```python
from build123d import *

# Parameters (mm, degrees)
ACTUATOR_HOUSING_MOUNT_R    = 64.3
ACTUATOR_HOUSING_MOUNT_R_2  = 55.8
ACTUATOR_HOUSING_MOUNT_R_3  = 1.6
ACTUATOR_HOUSING_WALL_DEPTH = 25
SKETCH2_R                   = 64.3
SKETCH2_R_2                 = 1.6
SKETCH2_R_3                 = 55.8
BOSS_EXTRUDE2_DEPTH         = 5
CUT_EXTRUDE1_START          = -5
SKETCH3_R                   = 11.45
CUT_EXTRUDE1_DEPTH          = 4
SKETCH4_R                   = 11
CUT_EXTRUDE2_DEPTH          = 4
BOSS_EXTRUDE3_START         = 8
SKETCH6_R                   = 64.3
SKETCH6_R_2                 = 63.1
BOSS_EXTRUDE3_DEPTH         = 8
SKETCH7_R                   = 1.95
M3_INSERT_L12_DEPTH         = 12
CHAMFER2_SIZE               = 0.5
SKETCH9_R                   = 1.95
CUT_EXTRUDE5_DEPTH          = 10


with BuildPart() as part:
    # Actuator Housing Mount → Actuator Housing Wall (new body)
    with BuildSketch(Plane.XY.offset(19)):
        Circle(ACTUATOR_HOUSING_MOUNT_R)
        Circle(ACTUATOR_HOUSING_MOUNT_R_2, mode=Mode.SUBTRACT)
        with Locations((57.375994082, 15.373851279)):
            Circle(ACTUATOR_HOUSING_MOUNT_R_3, mode=Mode.SUBTRACT)
        with Locations((57.375994082, -15.373851279)):
            Circle(ACTUATOR_HOUSING_MOUNT_R_3, mode=Mode.SUBTRACT)
        with Locations((42.002142802, -42.002142802)):
            Circle(ACTUATOR_HOUSING_MOUNT_R_3, mode=Mode.SUBTRACT)
        with Locations((15.373851279, -57.375994082)):
            Circle(ACTUATOR_HOUSING_MOUNT_R_3, mode=Mode.SUBTRACT)
        with Locations((-15.373851279, -57.375994082)):
            Circle(ACTUATOR_HOUSING_MOUNT_R_3, mode=Mode.SUBTRACT)
        with Locations((-42.002142802, -42.002142802)):
            Circle(ACTUATOR_HOUSING_MOUNT_R_3, mode=Mode.SUBTRACT)
        with Locations((-57.375994082, -15.373851279)):
            Circle(ACTUATOR_HOUSING_MOUNT_R_3, mode=Mode.SUBTRACT)
        with Locations((-57.375994082, 15.373851279)):
            Circle(ACTUATOR_HOUSING_MOUNT_R_3, mode=Mode.SUBTRACT)
        with Locations((-42.002142802, 42.002142802)):
            Circle(ACTUATOR_HOUSING_MOUNT_R_3, mode=Mode.SUBTRACT)
        with Locations((-15.373851279, 57.375994082)):
            Circle(ACTUATOR_HOUSING_MOUNT_R_3, mode=Mode.SUBTRACT)
        with Locations((15.373851279, 57.375994082)):
            Circle(ACTUATOR_HOUSING_MOUNT_R_3, mode=Mode.SUBTRACT)
        with Locations((42.002142802, 42.002142802)):
            Circle(ACTUATOR_HOUSING_MOUNT_R_3, mode=Mode.SUBTRACT)
    extrude(amount=-ACTUATOR_HOUSING_WALL_DEPTH)

    # Sketch2 → Boss-Extrude2 (add)
    # profile 1 of 2: a face of its own
    with BuildSketch(Plane(origin=(0, 0, -6), x_dir=(-1, 0, 0), z_dir=(0, 0, -1))):
        with Locations(Location((0, 0, 0), (0, 0, 180))):
            Circle(SKETCH2_R)
        with Locations(Location((-15.373851279, 57.375994082, 0), (0, 0, 180))):
            Circle(SKETCH2_R_2, mode=Mode.SUBTRACT)
        with Locations(Location((42.002142802, 42.002142802, 0), (0, 0, 180))):
            Circle(SKETCH2_R_2, mode=Mode.SUBTRACT)
        with Locations(Location((57.375994082, -15.373851279, 0), (0, 0, 180))):
            Circle(SKETCH2_R_2, mode=Mode.SUBTRACT)
        with Locations(Location((15.373851279, -57.375994082, 0), (0, 0, 180))):
            Circle(SKETCH2_R_2, mode=Mode.SUBTRACT)
        with Locations(Location((-42.002142802, -42.002142802, 0), (0, 0, 180))):
            Circle(SKETCH2_R_2, mode=Mode.SUBTRACT)
        with Locations(Location((-57.375994082, -15.373851279, 0), (0, 0, 180))):
            Circle(SKETCH2_R_2, mode=Mode.SUBTRACT)
        with Locations(Location((-57.375994082, 15.373851279, 0), (0, 0, 180))):
            Circle(SKETCH2_R_2, mode=Mode.SUBTRACT)
        with Locations(Location((0, 0, 0), (0, 0, 180))):
            Circle(SKETCH2_R_3, mode=Mode.SUBTRACT)
        with Locations(Location((-15.373851279, -57.375994082, 0), (0, 0, 180))):
            Circle(SKETCH2_R_2, mode=Mode.SUBTRACT)
        with Locations(Location((42.002142802, -42.002142802, 0), (0, 0, 180))):
            Circle(SKETCH2_R_2, mode=Mode.SUBTRACT)
        with Locations(Location((57.375994082, 15.373851279, 0), (0, 0, 180))):
            Circle(SKETCH2_R_2, mode=Mode.SUBTRACT)
        with Locations(Location((15.373851279, 57.375994082, 0), (0, 0, 180))):
            Circle(SKETCH2_R_2, mode=Mode.SUBTRACT)
        with Locations(Location((-42.002142802, 42.002142802, 0), (0, 0, 180))):
            Circle(SKETCH2_R_2, mode=Mode.SUBTRACT)
    # profile 2 of 2: a face of its own
    with BuildSketch(Plane(origin=(0, 0, -6), x_dir=(-1, 0, 0), z_dir=(0, 0, -1))):
        with Locations(Location((0, 0, 0), (0, 0, 180))):
            Circle(SKETCH2_R_3)
    extrude(amount=BOSS_EXTRUDE2_DEPTH)

    # Sketch3 → Cut-Extrude1 (cut)
    with BuildSketch(Plane(origin=(0, 0, -11), x_dir=(-1, 0, 0), z_dir=(0, 0, -1)).offset(CUT_EXTRUDE1_START)):
        Circle(SKETCH3_R)
    extrude(amount=CUT_EXTRUDE1_DEPTH, mode=Mode.SUBTRACT)

    # Sketch4 → Cut-Extrude2 (cut)
    with BuildSketch(Plane(origin=(0, 0, -11), x_dir=(-1, 0, 0), z_dir=(0, 0, -1))):
        Circle(SKETCH4_R)
    extrude(amount=-CUT_EXTRUDE2_DEPTH, mode=Mode.SUBTRACT)

    # Sketch6 → Boss-Extrude3 (add)
    with BuildSketch(Plane.XY.offset(19).offset(BOSS_EXTRUDE3_START)):
        Circle(SKETCH6_R)
        Circle(SKETCH6_R_2, mode=Mode.SUBTRACT)
    extrude(amount=-BOSS_EXTRUDE3_DEPTH)

    # Sketch7 → M3 Insert L12 (cut)
    with BuildSketch(Plane.XY.offset(19)):
        with Locations((57.375994082, -15.373851279)):
            Circle(SKETCH7_R)
        with Locations((42.002142802, -42.002142802)):
            Circle(SKETCH7_R)
        with Locations((15.373851279, -57.375994082)):
            Circle(SKETCH7_R)
        with Locations((-15.373851279, -57.375994082)):
            Circle(SKETCH7_R)
        with Locations((-42.002142802, -42.002142802)):
            Circle(SKETCH7_R)
        with Locations((-57.375994082, -15.373851279)):
            Circle(SKETCH7_R)
        with Locations((-57.375994082, 15.373851279)):
            Circle(SKETCH7_R)
        with Locations((-42.002142802, 42.002142802)):
            Circle(SKETCH7_R)
        with Locations((-15.373851279, 57.375994082)):
            Circle(SKETCH7_R)
        with Locations((15.373851279, 57.375994082)):
            Circle(SKETCH7_R)
        with Locations((42.002142802, 42.002142802)):
            Circle(SKETCH7_R)
        with Locations((57.375994082, 15.373851279)):
            Circle(SKETCH7_R)
    extrude(amount=-M3_INSERT_L12_DEPTH, mode=Mode.SUBTRACT)

    # Chamfer2
    chamfer2_edges = [part.edges().sort_by_distance(p)[0] for p in [
        (-64.3, 0, 27),
        (-64.3, 0, -11),
    ]]
    chamfer(chamfer2_edges, length=CHAMFER2_SIZE)

    # Sketch9 → Cut-Extrude5 (cut)
    with BuildSketch(Plane(origin=(0, 0, -11), x_dir=(-1, 0, 0), z_dir=(0, 0, -1))):
        with Locations((-30, 22)):
            Circle(SKETCH9_R)
        with Locations((30, 22)):
            Circle(SKETCH9_R)
        with Locations((30, -22)):
            Circle(SKETCH9_R)
        with Locations((-30, -22)):
            Circle(SKETCH9_R)
    extrude(amount=-CUT_EXTRUDE5_DEPTH, mode=Mode.SUBTRACT)


solid = part.part
```
Build history of the part. All positions in model axes, mm. A direction names the side the tool comes from. Round coordinates to 2 decimals unless told otherwise and drop trailing zeros. Write each loop counter-clockwise with the first axis right and the second up, starting at its lowest first coordinate (ties: lowest second). Pieces come first, ordered by that corner, then holes.
1) Band-saw the part on A-A, the plane y = 0. List the corners of the cut face in (x, z).
2) 3-axis set-ups, long thin cutter, end or side, ignore diameter. For faces 1 (the cylindrical face through (-57.58, -16.96, -1.87)), 2 (the cylindrical face through (-55.516, -14.788, 13.084)): which of +Z, -Z, +X, -X, +Y, -Y reach the whole face in a straight line?
3) Band-saw the part on C-C, the plane z = 14. Give the number of separate pieces and of enclosed holes in the cut face, and give its area (3 significant figures).
4) Mould opens along Y. For faces 3 (the flat face through (13, -1, -11)), 4 (the flat face through (-1, 12, -6)) say: +Y half, -Y half, draft (parallel to the pull), parting line (faces both ways), or undercut.
5) Drill centre lines: probe 1 along Y at (x, z) = (1, 25.5); probe 2 along Z at (x, y) = (-5.5, 37); probe 3 along Y at (x, z) = (31, -5). Where is each one in solid material? Low to high.
6) Pin check, flat tips, straight feed: pin 1 (5 mm diameter, centred on x = -57.38, y = -15.37, fed in from +Z); pin 2 (8 mm diameter, centred on y = -32, z = -7, fed in from +X); pin 3 (2.5 mm diameter, centred on x = 15.37, y = 57.38, fed in from -Z); pin 4 (3 mm diameter, centred on x = 18, z = 22, fed in from -Y). Stop position of each tip, or through.
Ans:
1. outline: (-64.3, -10.5) - (-63.8, -11) - (-11, -11) - (-11, -10) - (-11.45, -10) - (-11.45, -6) - (-55.8, -6) - (-55.8, 19) - (-63.1, 19) - (-63.1, 27) - (-63.8, 27) - (-64.3, 26.5) - close; (11, -11) - (63.8, -11) - (64.3, -10.5) - (64.3, 26.5) - (63.8, 27) - (63.1, 27) - (63.1, 19) - (55.8, 19) - (55.8, -6) - (11.45, -6) - (11.45, -10) - (11, -10) - close
2. face 1: +Z, -Z
2. face 2: +Z
3. separate pieces: 1
3. enclosed holes: 13
3. area: 3,060 mm2
4. face 3: draft
4. face 4: undercut
5. probe 1: y = -64.29 to -63.09, 63.09 to 64.29
5. probe 2: z = -11 to -6
5. probe 3: y = -56.33 to -46.4, 46.4 to 56.33
6. pin 1: stops at z = 19
6. pin 2: stops at x = 57.88
6. pin 3: passes through
6. pin 4: stops at y = -62.15
